```python
from build123d import *

# Parameters (mm, degrees)
F0_R        = 1.45
F1_DEPTH    = 27.5
F2_R        = 2.9
F3_DEPTH    = 1.8
F4_W        = 1
F4_H        = 1
F5_DEPTH    = 1.5
F6_S5_R     = 1.45
F6_T6_DEPTH = 6


# Not quite as in the source:
# - a fillet or chamfer that OpenCascade refuses, or shapes differently, is made with other operations: its cross-section is extruded or revolved along the edge and cut away or added


with BuildPart() as f1:
    # F0 (on Top) → F1 (new body)
    with BuildSketch(Plane.XY):
        Circle(F0_R)
    extrude(amount=F1_DEPTH)

    # F2 (on Top) → F3 (join)
    with BuildSketch(Plane.XY):
        Circle(F2_R)
    extrude(amount=-F3_DEPTH)

    # F4 (on face) → F5 (cut)
    with BuildSketch(Plane(origin=(0, 0, -1.8), x_dir=(1, 0, 0), z_dir=(0, 0, -1))):
        with Locations((1, 0)):
            Rectangle(F4_W, F4_H)
        Rectangle(F4_W, F4_H)
        with Locations((0, 1)):
            Rectangle(F4_W, F4_H)
        with Locations((-1, 0)):
            Rectangle(F4_W, F4_H)
        with Locations((0, -1)):
            Rectangle(F4_W, F4_H)
    extrude(amount=-F5_DEPTH, mode=Mode.SUBTRACT)

    # F6: chamfer of 1.5 on 1 edges, made by hand


with BuildPart() as f6_tool2:
    # F6_s3 → F6_t4 (revolve)
    with BuildSketch(Plane.XZ):
        Polygon((2.9, -1.5), (1.4, 0), (2.9, 0), align=None)
    revolve(axis=Axis((0, 0, 0), (0, 0, 1)))

    # F6_s5 → F6_t6 (cut, symmetric)
    with BuildSketch(Plane.XY.offset(-0.7)):
        Circle(F6_S5_R)
    extrude(amount=F6_T6_DEPTH, both=True, mode=Mode.SUBTRACT)


with BuildPart() as f1_1:
    add(f1.part)

    # F6_t1: cut F6_tool2
    add(f6_tool2.part, mode=Mode.SUBTRACT)


solid = f1_1.part
```
The listing builds one solid part. Answer for the finished solid, in the listing's coordinates (mm). A direction names the side the tool comes from. Give positions to 0.01 mm unless a question says otherwise; leave off trailing zeros. Order: outer loops, then holes, each group sorted by start corner. A loop starts at its lowest first (then second) coordinate and runs counter-clockwise, first axis right, second up.
Item 1: The part is cut by section A-A, the plane y = 0. Give the vertices of the cut face in (x, z).
From the geometry:
outline: (-2.9, -1.8) - (-1.5, -1.8) - (-1.5, -0.3) - (1.5, -0.3) - (1.5, -1.8) - (2.9, -1.8) - (2.9, -1.5) - (1.45, -0.05) - (1.45, 27.5) - (-1.45, 27.5) - (-1.45, -0.05) - (-2.9, -1.5) - close
Item 2: Given pin 1 Ø1.1 at (y, z) = (-1, -0.5) entering from +X; pin 2 Ø3 at (x, z) = (0.5, 21) entering from +Y; pin 3 Ø1.1 at (y, z) = (1, -1.5) entering from -X, each flat-ended and moving along its own axis, determine where each tip first touches the part or whether it passes through.
From the geometry:
pin 1: stops at x = 2.28
pin 2: stops at y = 1.45
pin 3: stops at x = -2.86
Item 3: Which of the six approach directions +Z, -Z, +X, -X, +Y, -Y give full straight-line access (tool end or side, diameter ignored) to faces 1 (the face through (-2.14, 1.96, -1.65)), 2 (the face through (0, -1.5, -1))?
From the geometry:
face 1: +Z, -Z
face 2: -Z
Item 4: Find the intervals of material crossed by probe 1 along X at (y, z) = (-0.1, 18.25); probe 2 along Z at (x, y) = (-1.95, -2.05), in increasing order.
From the geometry:
probe 1: x = -1.45 to 1.45
probe 2: z = -1.8 to -1.43
Item 5: For a pull along Z with two mould halves and no side action, classify faces 3 (the face through (-1.45, 0.06, 13.92)), 4 (the face through (1, -1, -1.8)), 5 (the face through (0, 0, 27.5)) as pulls with the +Z half, pulls with the -Z half, needs draft (parallel to the pull), parting line crosses it, or undercut.
From the geometry:
face 3: needs draft
face 4: pulls with the -Z half
face 5: pulls with the +Z half
Item 6: The part is cut by section C-C, the plane z = 19.75. Give the vertices of the cut face in (x, y), and give its area (3 significant figures).
From the geometry:
outline: circle Ø2.9 at (0, 0)
area: 6.61 mm2
